Input: part model. Units: mm. Frame: model coordinates. Face numbers are marked on the shaded views. A direction names the side the tool comes from. Round coordinates to 2 decimals unless told otherwise and drop trailing zeros. Order: outer loops, then holes, each group sorted by start corner. A loop starts at its lowest first (then second) coordinate and runs counter-clockwise, first axis right, second up.
Item 1: First-contact query: pin 1 (12 mm diameter, centred on x = -13, y = -48, fed in from +Z); pin 2 (16 mm diameter, centred on x = -725, y = 350, fed in from -Z). Flat tips, straight axial feed; report the tip coordinate or a pass-through.
Item 2: Mould query, pull axis X, two halves, no side actions, for the marked faces 3, 4 and 5. Classes: released by +X, released by -X, zero draft, split by the parting line, or undercut.
Item 3: Line query: L1, parallel to Y at x = 71.5, z = 80; L2, parallel to X at y = -296.5, z = 84.5; L3, parallel to Y at x = 725, z = 24. Output: solid intervals per line, ascending.
Item 4: Cut plane B-B on x = -650. Output: boundary loops of the cut face in (y, z), then the cut area to 3 significant figures.
Item 5: Cut plane A-A on z = 30. Give the number of separate pieces and of enclosed holes in the cut face, then the cut area to 3 significant figures.
Item 6: Cut plane C-C on y = 0. Output: boundary loops of the cut face in (x, z), then the cut area to 3 significant figures.
Item 7: Reachability of the marked faces 1 and 2 from +Z, -Z, +X, -X, +Y, -Y: full face, straight path, thin tool, end or side. Return the list, or none.
Item 8: Cut plane D-D on x = -447.5. Output: boundary loops of the cut face in (y, z), then the cut area to 3 significant figures.
```python
from build123d import *

# Parameters (mm, degrees)
SKETCH1_W                 = 1492
SKETCH1_H                 = 742
BOSS_EXTRUDE1_DEPTH       = 102
HOLE1_D                   = 10.1
HOLE1_DEPTH               = 102
HOLE1_CBORE_D             = 20.5
HOLE1_CBORE_DEPTH         = 2
M45_CLEARANCE_HOLE1_D     = 50
M45_CLEARANCE_HOLE1_DEPTH = 102
SHELL1_T                  = -3


with BuildPart() as part:
    # Sketch1 → Boss-Extrude1 (new body)
    with BuildSketch(Plane.XY.offset(102)):
        Rectangle(SKETCH1_W, SKETCH1_H)
    extrude(amount=-BOSS_EXTRUDE1_DEPTH)

    # Hole1
    with Locations(Plane(origin=(0, 0, 0), x_dir=(-1, 0, 0), z_dir=(0, 0, -1))):
        with Locations((725, 350), (-725, 350), (-725, -350), (725, -350), (0, 350), (0, -350)):
            CounterBoreHole(HOLE1_D / 2, HOLE1_CBORE_D / 2, HOLE1_CBORE_DEPTH, depth=HOLE1_DEPTH)

    # M45 Clearance Hole1
    with Locations(Plane.XY.offset(102)):
        with Locations((650, 50), (0, 0), (-650, 50)):
            Hole(M45_CLEARANCE_HOLE1_D / 2, depth=M45_CLEARANCE_HOLE1_DEPTH)

    # Shell1
    shell1_openings = [part.faces().sort_by_distance(p)[0] for p in [
        (675, 50, 102),
    ]]
    offset(amount=SHELL1_T, openings=shell1_openings, kind=Kind.INTERSECTION)


solid = part.part
```
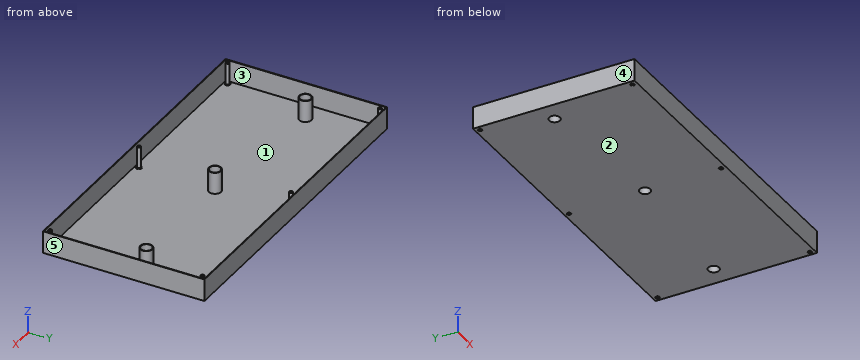
From the geometry:
1. pin 1: stops at z = 3
1. pin 2: stops at z = 2
2. face 3: undercut
2. face 4: released by -X
2. face 5: released by +X
3. L1: y = -371 to -368, 368 to 371
3. L2: x = -746 to -743, 743 to 746
3. L3: y = -371 to -368, -358.05 to -355.05, -344.95 to -341.95, 341.95 to 344.95, 355.05 to 358.05, 368 to 371
4. outline: (-371, 0) - (25, 0) - (25, 102) - (22, 102) - (22, 3) - (-368, 3) - (-368, 102) - (-371, 102) - close; (75, 0) - (371, 0) - (371, 102) - (368, 102) - (368, 3) - (78, 3) - (78, 102) - (75, 102) - close
4. area: 3,260 mm2
5. separate pieces: 10
5. enclosed holes: 10
5. area: 15,600 mm2
6. outline: (-746, 0) - (-25, 0) - (-25, 102) - (-28, 102) - (-28, 3) - (-743, 3) - (-743, 102) - (-746, 102) - close; (25, 0) - (746, 0) - (746, 102) - (743, 102) - (743, 3) - (28, 3) - (28, 102) - (25, 102) - close
6. area: 5,510 mm2
7. face 1: +Z
7. face 2: -Z, +X, -X, +Y, -Y
8. outline: (-371, 0) - (371, 0) - (371, 102) - (368, 102) - (368, 3) - (-368, 3) - (-368, 102) - (-371, 102) - close
8. area: 2,820 mm2
